```python
from build123d import *

# Parameters (mm, degrees)
F0_W      = 76.2
F0_H      = 24.6256076701
F1_DEPTH  = 38.1
F0_W_2    = 38.1
F0_H_2    = 25.4
F2_DEPTH  = 25.4
F2_FACE_W = 38.1
F2_FACE_H = 50.8
F3_ANGLE  = 60


with BuildPart() as f1:
    # F0 (on Front) → F1 (new body, symmetric)
    with BuildSketch(Plane.XZ):
        with Locations((-0.260655035, 0)):
            Rectangle(F0_W, F0_H)
    extrude(amount=F1_DEPTH, both=True)

    # F0 (on Front) → F2 (join, symmetric)
    with BuildSketch(Plane.XZ):
        with Locations((-0.260655035, 0)):
            Rectangle(F0_W, F0_H)
        Polygon((-38.360655035, 12.3128038351), (37.839344965, 12.3128038351), (39.9018798504, 64.5671242428), (1.8018798504, 64.5671242428), align=None)
        with Locations((20.8518798504, 77.2671242428)):
            Rectangle(F0_W_2, F0_H_2)
    extrude(amount=F2_DEPTH, both=True)

    # F2_face (on face) → F3 (revolve)
    with BuildSketch(Plane(origin=(20.8518798504, 0, 89.9671242428), x_dir=(1, 0, 0), z_dir=(0, 0, 1))):
        Rectangle(F2_FACE_W, F2_FACE_H)
    revolve(axis=Axis((39.9018798504, 0, 89.9671242428), (0, 1, 0)), revolution_arc=F3_ANGLE)


solid = f1.part
```
Work out the finished part from the listing and answer in its coordinate system (mm). A direction names the side the tool comes from. Round coordinates to 2 decimals unless told otherwise and drop trailing zeros. Write each loop counter-clockwise with the first axis right and the second up, starting at its lowest first coordinate (ties: lowest second). Pieces come first, ordered by that corner, then holes.
1) A cutting plane is placed at D-D on x = 16. Determine the outline of the cut face in (y, z).
2) A cutting plane is placed at C-C on z = 73. Determine the outline of the cut face in (x, y), and give its area (3 significant figures).
3) Which of the six approach directions +Z, -Z, +X, -X, +Y, -Y give full straight-line access (tool end or side, diameter ignored) to faces 1 (the face through (19, -25.4, 56)), 2 (the face through (37.839, -1, 0)), 3 (the face through (30.24, 0.36, 106.7)), 4 (the face through (1.802, 0, 77)), 5 (the face through (19, 25.4, 56))?
4) A cutting plane is placed at B-B on x = -10.5. Determine the outline of the cut face in (y, z).
5) Flat-ended cylindrical pins translate along their axes: P1, Ø1, axis at x = 13.5, y = -2.5, coming from the +Z side; P2, Ø23.5, axis at x = 9.5, z = 41.5, coming from the -Y side; P3, Ø10, axis at x = 20, z = 59, coming from the +Y side. Find the tip coordinate at first contact, or state that the pin passes through.
6) Consider probe 1 along Y at (x, z) = (-6, 25); probe 2 along X at (y, z) = (1.5, 71.5); probe 3 along Z at (x, y) = (-12.5, -26.5). Determine where each line is inside the solid, lowest interval first.
7) A cutting plane is placed at A-A on y = 11.5. Determine the outline of the cut face in (x, z), and give its area (3 significant figures).
Entries:
1. outline: (-38.1, -12.31) - (38.1, -12.31) - (38.1, 12.31) - (25.4, 12.31) - (25.4, 119.64) - (-25.4, 119.64) - (-25.4, 12.31) - (-38.1, 12.31) - close
2. outline: (1.8, -25.4) - (39.9, -25.4) - (39.9, 25.4) - (1.8, 25.4) - close
2. area: 1,940 mm2
3. face 1: +Z, +X, -X, -Y
3. face 2: -Z, +X, +Y, -Y
3. face 3: +Z, +X, +Y, -Y
3. face 4: +Z, -X, +Y, -Y
3. face 5: +Z, +X, -X, +Y
4. outline: (-38.1, -12.31) - (38.1, -12.31) - (38.1, 12.31) - (25.4, 12.31) - (25.4, 48.56) - (-25.4, 48.56) - (-25.4, 12.31) - (-38.1, 12.31) - close
5. P1: stops at z = 117.91
5. P2: stops at y = -25.4
5. P3: stops at y = 25.4
6. probe 1: y = -25.4 to 25.4
6. probe 2: x = 1.8 to 39.9
6. probe 3: z = -12.31 to 12.31
7. outline: (-38.36, -12.31) - (37.84, -12.31) - (37.84, 12.31) - (39.9, 64.57) - (39.9, 89.97) - (20.85, 122.96) arc R38.1 ccw to (1.8, 89.97) - (1.8, 64.57) - (-38.36, 12.31) - close
7. area: 6,590 mm2
